```python
from build123d import *

# Parameters (mm, degrees)
SKETCH2_W              = 18
SKETCH2_H              = 4
M3_TAPPED_HOLE1_REACH  = 24.45
M3_TAPPED_HOLE1_BORE_R = 1.25
M3_TAPPED_HOLE2_REACH  = 24.45
M3_TAPPED_HOLE2_BORE_R = 1.25


with BuildPart() as part:
    # Sketch2 → Revolve1 (revolve)
    with BuildSketch(Plane.XY, mode=Mode.PRIVATE) as revolve1_sk:
        with Locations((9, 4)):
            Rectangle(SKETCH2_W, SKETCH2_H)
    revolve(revolve1_sk.sketch.rotate(Axis((0, 0, 0), (1, 0, 0)), 90), axis=Axis((0, 0, 0), (1, 0, 0)))

    # M3 Tapped Hole1 bore → M3 Tapped Hole1 (cut, up to next)
    with BuildSketch(Plane(origin=(0, -6, 0), x_dir=(-1, 0, 0), z_dir=(0, -1, 0)), mode=Mode.PRIVATE) as m3_tapped_hole1_sk1:
        with Locations((-15.5, 0)):
            Circle(M3_TAPPED_HOLE1_BORE_R)
    m3_tapped_hole1_tool1 = extrude(m3_tapped_hole1_sk1.sketch, amount=-M3_TAPPED_HOLE1_REACH, mode=Mode.PRIVATE) & part.part
    # M3 Tapped Hole1 bore → M3 Tapped Hole1 (cut, up to next)
    with BuildSketch(Plane(origin=(0, -6, 0), x_dir=(-1, 0, 0), z_dir=(0, -1, 0)), mode=Mode.PRIVATE) as m3_tapped_hole1_sk2:
        with Locations((-2.5, 0)):
            Circle(M3_TAPPED_HOLE1_BORE_R)
    m3_tapped_hole1_tool2 = extrude(m3_tapped_hole1_sk2.sketch, amount=-M3_TAPPED_HOLE1_REACH, mode=Mode.PRIVATE) & part.part
    add(m3_tapped_hole1_tool1.solids().sort_by_distance((15.5, -6, 0))[0], mode=Mode.SUBTRACT)
    add(m3_tapped_hole1_tool2.solids().sort_by_distance((2.5, -6, 0))[0], mode=Mode.SUBTRACT)

    # M3 Tapped Hole2 bore → M3 Tapped Hole2 (cut, up to next)
    with BuildSketch(Plane.XY.offset(6), mode=Mode.PRIVATE) as m3_tapped_hole2_sk1:
        with Locations((2.5, 0)):
            Circle(M3_TAPPED_HOLE2_BORE_R)
    m3_tapped_hole2_tool1 = extrude(m3_tapped_hole2_sk1.sketch, amount=-M3_TAPPED_HOLE2_REACH, mode=Mode.PRIVATE) & part.part
    # M3 Tapped Hole2 bore → M3 Tapped Hole2 (cut, up to next)
    with BuildSketch(Plane.XY.offset(6), mode=Mode.PRIVATE) as m3_tapped_hole2_sk2:
        with Locations((15.5, 0)):
            Circle(M3_TAPPED_HOLE2_BORE_R)
    m3_tapped_hole2_tool2 = extrude(m3_tapped_hole2_sk2.sketch, amount=-M3_TAPPED_HOLE2_REACH, mode=Mode.PRIVATE) & part.part
    add(m3_tapped_hole2_tool1.solids().sort_by_distance((2.5, 0, 6))[0], mode=Mode.SUBTRACT)
    add(m3_tapped_hole2_tool2.solids().sort_by_distance((15.5, 0, 6))[0], mode=Mode.SUBTRACT)


solid = part.part
```
Verification items for the finished model (mm, model axes). A direction names the side the tool comes from. Give positions to 0.01 mm unless a question says otherwise; leave off trailing zeros. Write each loop counter-clockwise with the first axis right and the second up, starting at its lowest first coordinate (ties: lowest second). Pieces come first, ordered by that corner, then holes. Notation, with made-up numbers: M 48,1.5 L 53,1.5 A12 ccw 53,22.5 Z; hole C 40,24.5 d2. An arc over 180 degrees is marked long. One line per question, with ' | ' between items.
1) Mould release check, pull along Z, two halves, no side actions. Record for faces 4 (the cylindrical face through (15.66, -3.81, -1.24)), 5 (the cylindrical face through (9.126, 5.857, -1.301)), 6 (the flat face through (0, 0, -3)): released by +Z, released by -Z, zero draft, split by the parting line, or undercut.
Result:
face 4: undercut | face 5: split by the parting line | face 6: zero draft
2) Gauge pin test, flat ends, axial feed: pin 1 Ø3.5 at (y, z) = (0, 0) entering from +X; pin 2 Ø2 at (x, y) = (2.5, 0) entering from +Z; pin 3 Ø4 at (x, y) = (8.5, -3) entering from -Z; pin 4 Ø2 at (x, z) = (10, -1.5) entering from +Y. Record the tip position at first contact, or that the pin passes through.
Result:
pin 1: passes through | pin 2: stops at z = -1.73 | pin 3: stops at z = -5.92 | pin 4: stops at y = 5.98
3) Section check B-B on x = 15.5. Enter the section's corners in (y, z), plus the area to 3 significant figures.
Result:
outline: M -5.87,-1.25 A6 ccw long 1.25,5.87 L 1.25,1.56 A2 cw long -1.56,-1.25 Z; M -5.87,1.25 L -1.56,1.25 A2 cw -1.25,1.56 L -1.25,5.87 A6 ccw Z | area: 80.1 mm2
4) Section check A-A on z = 0. Enter the section's corners in (x, y).
Result:
outline: M 0,-6 L 1.25,-6 L 1.25,-2 L 0,-2 Z; M 0,2 L 18,2 L 18,6 L 0,6 Z; M 3.75,-6 L 14.25,-6 L 14.25,-2 L 3.75,-2 Z; M 16.75,-6 L 18,-6 L 18,-2 L 16.75,-2 Z
5) Section check C-C on y = 0. Enter the section's corners in (x, z), plus the area to 3 significant figures.
Result:
outline: M 0,-6 L 18,-6 L 18,-2 L 0,-2 Z; M 0,2 L 1.25,2 L 1.25,6 L 0,6 Z; M 3.75,2 L 14.25,2 L 14.25,6 L 3.75,6 Z; M 16.75,2 L 18,2 L 18,6 L 16.75,6 Z | area: 124 mm2
6) Thickness scan on line 1 along X through (y, z) = (-3.5, 0); line 2 along Y through (x, z) = (13.5, 0); line 3 along X through (y, z) = (-0.75, 5.5). Record the ranges inside material, lowest first. Write a range as [from, to].
Result:
line 1: x = [0, 1.25], [3.75, 14.25], [16.75, 18] | line 2: y = [-6, -2], [2, 6] | line 3: x = [0, 1.5], [3.5, 14.5], [16.5, 18]
7) Set-up check for faces 1 (the cylindrical face through (15.34, 1.24, 3.81)), 2 (the flat face through (18, 0, -3)), 3 (the cylindrical face through (2.66, -3.81, -1.24)): record each of +Z, -Z, +X, -X, +Y, -Y from which the full face is reachable in a straight line by a thin tool's end or side.
Result:
face 1: +Z | face 2: +Z, -Z, +X, +Y, -Y | face 3: -Y
8) Section check D-D on x = 6. Enter the section's corners in (y, z), plus the area to 3 significant figures.
Result:
outline: C 0,0 d12; hole C 0,0 d4 | area: 101 mm2
